from build123d import *

# Parameters (mm, degrees)
SKETCH_1_R          = 10
EXTRUDE_1_DEPTH     = 24
M3X0_52_D           = 2.5
M3X0_52_DEPTH       = 8.5
M3X0_52_TIP         = 0.751075774
EXTRUDE_START       = 3
SKETCH_10_R         = 11.5
SKETCH_10_R_2       = 10
EXTRUDE_2_DEPTH     = 3
SKETCH_8_R          = 10
SKETCH_8_R_2        = 9.5
CUT_EXTRUDE_1_DEPTH = 1.3


with BuildPart() as part:
    # Эскиз1 → Бобышка-Вытянуть1 (new body)
    with BuildSketch(Plane(origin=(0, 0, 0), x_dir=(1, 0, 0), z_dir=(0, 1, 0))):
        with Locations(Location((0, 0, 0), (0, 0, 270))):
            Circle(SKETCH_1_R)
    extrude(amount=EXTRUDE_1_DEPTH)

    # Отверстие обработанное метчиком M3x0.52
    with Locations(Plane(origin=(-4.838819278, 24, -4.760025704), x_dir=(-1, 0, 0), z_dir=(0, 1, 0))):
        with Locations((-4.838819278, -1.239974296), (-10.838819278, 4.760025704), (-4.838819278, 10.760025704), (1.161180722, 4.760025704)):
            Hole(M3X0_52_D / 2, depth=M3X0_52_DEPTH)
            with Locations((0, 0, -(M3X0_52_DEPTH + M3X0_52_TIP / 2))):  # 118° drill point
                Cone(0, M3X0_52_D / 2, M3X0_52_TIP, mode=Mode.SUBTRACT)

    # Эскиз10 → Бобышка-Вытянуть2 (add)
    with BuildSketch(Plane(origin=(0, 3, 0), x_dir=(-1, 0, 0), z_dir=(0, -1, 0)).offset(EXTRUDE_START)):
        with Locations(Location((0, 0, 0), (0, 0, 270))):
            Circle(SKETCH_10_R)
        with Locations(Location((0, 0, 0), (0, 0, 90))):
            Circle(SKETCH_10_R_2, mode=Mode.SUBTRACT)
    extrude(amount=-EXTRUDE_2_DEPTH)

    # Эскиз8 → Вырез-Вытянуть1 (cut)
    with BuildSketch(Plane(origin=(0, 13, 0), x_dir=(1, 0, 0), z_dir=(0, 1, 0))):
        with Locations(Location((0, 0, 0), (0, 0, 270))):
            Circle(SKETCH_8_R)
        with Locations(Location((0, 0, 0), (0, 0, 270))):
            Circle(SKETCH_8_R_2, mode=Mode.SUBTRACT)
    extrude(amount=CUT_EXTRUDE_1_DEPTH, mode=Mode.SUBTRACT)


solid = part.part
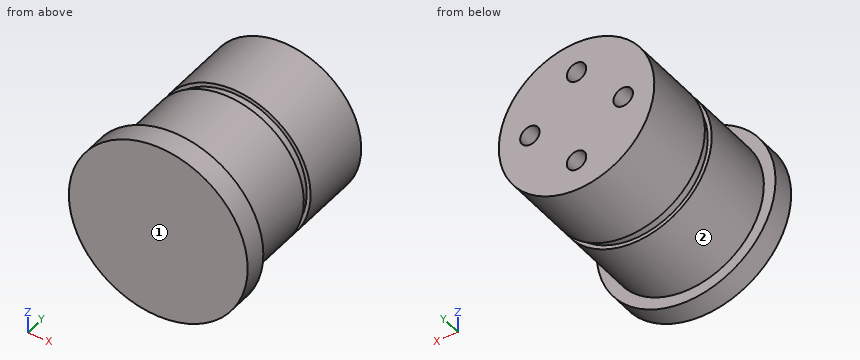
Build history of the part. All positions in model axes, mm. Face numbers are marked on the shaded views. A direction names the side the tool comes from. Give positions to 0.01 mm unless a question says otherwise; leave off trailing zeros. Write each loop counter-clockwise with the first axis right and the second up, starting at its lowest first coordinate (ties: lowest second). Pieces come first, ordered by that corner, then holes. Notation, with made-up numbers: (25, -2) - (57, -2) arc R35 ccw to (57, 37) - close; hole circle Ø3 at (-15, 39). An arc over 180 degrees is marked (long way). Use one line per item in the form item = value. Start each with the question number.
1. Drop flat-ended pins along their axis: pin 1 Ø2 at (y, z) = (7, -1.5) entering from -X; pin 2 Ø5 at (y, z) = (8.5, -7.5) entering from +X; pin 3 Ø3 at (x, z) = (0, 6) entering from +Y; pin 4 Ø1.5 at (x, z) = (-6, 0) entering from +Y. Give the stop position or say it passes through.
2. Band-saw the part on B-B on z = 8. Write the cut outline in (x, y).
3. Band-saw the part on C-C on x = 4.25. Write the cut outline in (y, z), plus the area to 3 significant figures.
4. 3-axis set-ups, long thin cutter, end or side, ignore diameter. For the marked faces 1 and 2: which of +Z, -Z, +X, -X, +Y, -Y reach the whole face in a straight line?
5. Probe line 1 (X direction, y = 19.75, z = 0); line 2 (Y direction, x = -8.5, z = 5); line 3 (X direction, y = 23, z = -7). List the from-to ranges inside material, lowest first. Write a range as [from, to].
6. Band-saw the part on D-D on y = 10.5. Write the cut outline in (x, z), plus the area to 3 significant figures.
7. Band-saw the part on A-A on y = 21. Write the cut outline in (x, z).
Conclusion:
q1.pin_1 = -9.99
q1.pin_2 = 8.66
q1.pin_3 = 24
q1.pin_4 = 15.2
q2.outline = (-8.26, 0) - (8.26, 0) - (8.26, 3) - (6, 3) - (6, 13) - (5.12, 13) - (5.12, 14.3) - (6, 14.3) - (6, 24) - (-6, 24) - (-6, 14.3) - (-5.12, 14.3) - (-5.12, 13) - (-6, 13) - (-6, 3) - (-8.26, 3) - close
q3.outline = (0, -10.69) - (3, -10.69) - (3, -9.05) - (13, -9.05) - (13, -8.5) - (14.3, -8.5) - (14.3, -9.05) - (24, -9.05) - (24, 9.05) - (14.3, 9.05) - (14.3, 8.5) - (13, 8.5) - (13, 9.05) - (3, 9.05) - (3, 10.69) - (0, 10.69) - close
q3.area = 443 mm²
q4.face_1 = +Z, -Z, +X, -X, -Y
q4.face_2 = +Y
q5.line_1 = [-10, -7.25], [-4.75, 4.75], [7.25, 10]
q5.line_2 = [0, 13], [14.3, 24]
q5.line_3 = [-7.14, -0.75], [0.75, 7.14]
q6.outline = circle Ø20 at (0, 0)
q6.area = 314 mm²
q7.outline = circle Ø20 at (0, 0); hole circle Ø2.5 at (-6, 0); hole circle Ø2.5 at (0, -6); hole circle Ø2.5 at (0, 6); hole circle Ø2.5 at (6, 0)
